Verification items for this drawing (mm, ordinates from the low corner). A direction names the side the tool comes from. Round coordinates to 2 decimals unless told otherwise and drop trailing zeros. Write each loop counter-clockwise with the first axis right and the second up, starting at its lowest first coordinate (ties: lowest second). Pieces come first, ordered by that corner, then holes. Notation, with made-up numbers: M -40,78.5 L -34,78.5 A32 cw -34,115.5 Z; hole C 86.25,-24 d3. An arc over 180 degrees is marked long. Write each question's results on one line, items separated by ' | '.
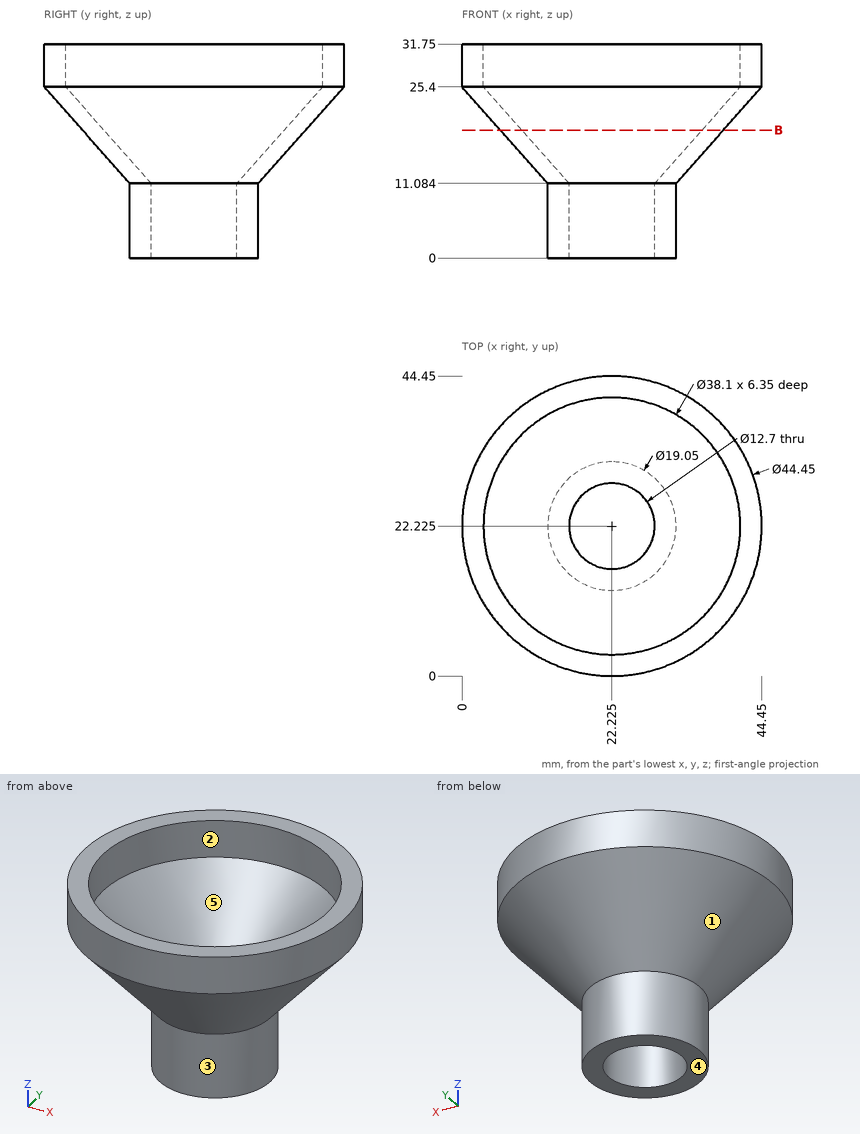
1) Depth check by flat-ended pin: P1, Ø16.5, axis at x = 22.225, y = 22.225, coming from the +Z side (1 decimal); P2, Ø4, axis at y = 32.5, z = 6.5, coming from the +X side; P3, Ø12, axis at x = 7.5, z = 24, coming from the +Y side (1 decimal). Enter the tip coordinate at first touch or a pass-through.
Calculated:
P1: stops at z = 13.2 | P2: stops at x = 26.94 | P3: stops at y = 42.6
2) Material ranges on line 1 (Y direction, x = 20.5, z = 10.5); line 2 (X direction, y = 30.5, z = 27) (1 decimal); line 3 (X direction, y = 21, z = 17), recorded low to high. Write a range as [from, to].
Calculated:
line 1: y = [12.86, 16.11], [28.34, 31.59] | line 2: x = [1.6, 5.1], [39.4, 42.9] | line 3: x = [7.5, 10.69], [33.76, 36.95]
3) Sectioned sample at B-B, the plane z = 19. Record the cut outline in (x, y) (1 decimal).
Calculated:
outline: C 22.2,22.2 d33.1; hole C 22.2,22.2 d26.7
4) Draft check along X on the marked faces 3, 4 and 5. Enter one of: pulls with the +X half, pulls with the -X half, needs draft (parallel to the pull), parting line crosses it, or undercut.
Calculated:
face 3: parting line crosses it | face 4: needs draft | face 5: undercut
5) Access from +Z, -Z, +X, -X, +Y, -Y to the whole of each face (thin tool, end or side, straight path). Record for the marked faces 1 and 2.
Calculated:
face 1: -Z | face 2: +Z
